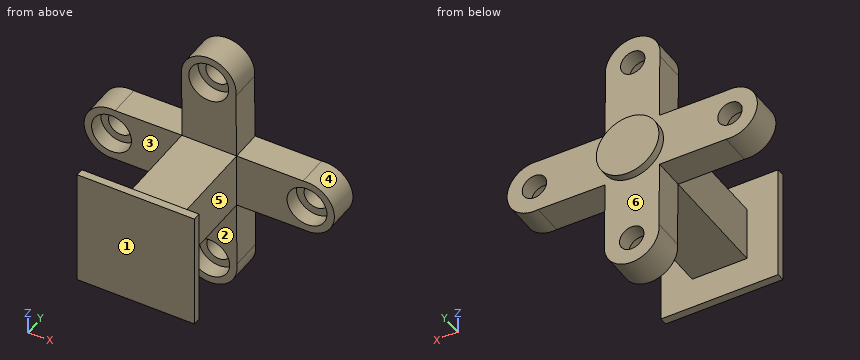
Autodesk Inventor part; units mm, degrees
ref_plane "YZ Plane" through (0, 0, 0) normal (1, 0, 0) x (0, 1, 0)
ref_plane "XZ Plane" through (0, 0, 0) normal (0, 1, 0) x (-1, 0, 0)
ref_plane "XY Plane" through (0, 0, 0) normal (0, 0, 1) x (1, 0, 0)
sketch "Sketch1" plane through (0, 0, 0) normal (0, 1, 0) x (-1, 0, 0)
  line L0 (5, 5) -> (-5, 5)
  line L1 (-5, 5) -> (-5, -5)
  line L2 (-5, -5) -> (5, -5)
  line L3 (5, -5) -> (5, 5)
  line L4 (5, 5) -> (-5, -5) construction
  line L5 (-5, 5) -> (5, -5) construction
  line L6 (-7, 7) -> (7, 7)
  line L7 (7, 7) -> (7, -7)
  line L8 (7, -7) -> (-7, -7)
  line L9 (-7, -7) -> (-7, 7)
  point P0 (0, 0)
  dimension "d0" = 10
  dimension "d1" = 10
  dimension "d4" = 2
extrude "Extrusion1" add sketch "Sketch1" along normal blind 29.7 contours L3 L2 L1 L0 | L6 L7 L8 L9
sketch "Sketch2" plane through (0, 29.7, 0) normal (0, 1, 0) x (1, 0, 0)
  circle A0 centre (0, 0) radius 25 construction
  circle A1 centre (0.126, 24.9997) radius 3.125
  arc A2 (7.0521, 23.9848) -> (-6.8099, 24.0546) centre (0.126, 24.9997) ccw
  line L0 (-7, 7) -> (-7, -7)
  line L1 (7, -7) -> (7, 7)
  line L2 (7, 7) -> (-7, 7) construction
  line L3 (-6.8099, 24.0546) -> (-7, 7)
  line L4 (7.0521, 23.9848) -> (7, 7)
  circle A3 centre (-24.9997, 0.126) radius 3.125
  arc A4 (-23.9848, 7.0521) -> (-24.0546, -6.8099) centre (-24.9997, 0.126) ccw
  line L5 (-23.9848, 7.0521) -> (-7, 7)
  line L6 (-24.0546, -6.8099) -> (-7, -7)
  circle A5 centre (-0.126, -24.9997) radius 3.125
  arc A6 (-7.0521, -23.9848) -> (6.8099, -24.0546) centre (-0.126, -24.9997) ccw
  line L7 (-7.0521, -23.9848) -> (-7, -7)
  line L8 (6.8099, -24.0546) -> (7, -7)
  circle A7 centre (24.9997, -0.126) radius 3.125
  arc A8 (23.9848, -7.0521) -> (24.0546, 6.8099) centre (24.9997, -0.126) ccw
  line L9 (23.9848, -7.0521) -> (7, -7)
  line L10 (24.0546, 6.8099) -> (7, 7)
  point P0 (7, 7)
  point P1 (-7, 7)
  point P2 (-7, -7)
  point P3 (7, -7)
  dimension "d5" = 50
  dimension "d6" = 6.25
  dimension "d10" = 360
  dimension "d28" = 7
extrude "Extrusion2" add sketch "Sketch2" along normal blind 8
sketch "Sketch3" plane through (0, 29.7, 0) normal (0, -1, 0) x (1, 0, 0)
  circle A0 centre (24.9997, 0.126) radius 3.125
  circle A1 centre (24.9997, 0.126) radius 5.1
  circle A2 centre (-0.126, 24.9997) radius 5.1
  circle A3 centre (-24.9997, -0.126) radius 5.1
  circle A4 centre (0.126, -24.9997) radius 5.1
  point P0 (0, 0)
  dimension "d14" = 10.2
  dimension "d17" = 360
extrude "Extrusion3" cut sketch "Sketch3" against normal blind 4
sketch "Sketch6" plane through (0, 0, 0) normal (0, -1, 0) x (1, 0, 0)
  line L0 (-15, -15) -> (15, -15)
  line L1 (15, -15) -> (15, 15)
  line L2 (15, 15) -> (-15, 15)
  line L3 (-15, 15) -> (-15, -15)
  line L4 (-15, -15) -> (15, 15) construction
  line L5 (15, -15) -> (-15, 15) construction
  point P0 (0, 0)
  dimension "d32" = 30
  dimension "d33" = 30
extrude "Extrusion4" add sketch "Sketch6" along normal blind 2
sketch "Sketch7" plane through (0, 37.7, 0) normal (0, 1, 0) x (1, 0, 0)
  circle A0 centre (0, 0) radius 8
  dimension "d36" = 16
extrude "Extrusion5" add sketch "Sketch7" along normal blind 2
equation "\"d1\" = d0"
properties part number "franka_mount_3DPrint"
CAD build for the part. Positions are in the model's coordinates, mm. Face numbers are marked on the shaded views. A direction names the side the tool comes from. Round coordinates to 2 decimals unless told otherwise and drop trailing zeros. Order: outer loops, then holes, each group sorted by start corner. A loop starts at its lowest first (then second) coordinate and runs counter-clockwise, first axis right, second up.
Q1. Two-plate mould, pull along Y, no slides. Class the marked faces 4, 5 and 6: pulls with the +Y half, pulls with the -Y half, needs draft (parallel to the pull), parting line crosses it, or undercut.
Q2. Drop flat-ended pins along their axis: pin 1 (11 mm diameter, centred on x = -23.5, z = -1, fed in from -Y); pin 2 (7 mm diameter, centred on x = -1.5, y = 15.5, fed in from +Z); pin 3 (10 mm diameter, centred on y = 6.5, z = 16, fed in from -X); pin 4 (11.5 mm diameter, centred on x = 2.5, z = -19, fed in from -Y). Give the stop position or say it passes through.
Q3. Slice it at A-A (z = -9.5). Write the cut outline in (x, y), and give its area (3 significant figures).
Q4. Wall check: L1, parallel to Z at x = -5.5, y = 8.5; L2, parallel to Y at x = 10.5, z = -0.5. Give the ranges that are in metal, low to high.
Q5. Which spindle directions (+Z, -Z, +X, -X, +Y, -Y) get a long thin tool onto all of the face, cutting with end or side? Do the marked faces 1, 2 and 3. Say none if no direction does.
Q6. Slice it at B-B (x = 0). State how many separate pieces and enclosed holes the cut face has, and give its area (3 significant figures).
Results below:
1. face 4: needs draft
1. face 5: undercut
1. face 6: pulls with the +Y half
2. pin 1: stops at y = 29.7
2. pin 2: stops at z = 7
2. pin 3: passes through
2. pin 4: stops at y = -2
3. outline: (-15, -2) - (15, -2) - (15, 0) - (-15, 0) - close; (-6.97, 29.7) - (7.01, 29.7) - (7.01, 37.7) - (-6.97, 37.7) - close
3. area: 172 mm2
4. L1: z = -7 to 7
4. L2: y = -2 to 0, 29.7 to 37.7
5. face 1: +Z, -Z, +X, -X, -Y
5. face 2: -Z, +X, -X
5. face 3: +Z, -Z, -X
6. separate pieces: 3
6. enclosed holes: 0
6. area: 888 mm2
